Geometry: final body of the model. Coordinates: model frame, mm. A direction names the side the tool comes from. Give positions to 0.01 mm unless a question says otherwise; leave off trailing zeros. Order: outer loops, then holes, each group sorted by start corner. A loop starts at its lowest first (then second) coordinate and runs counter-clockwise, first axis right, second up. Notation, with made-up numbers: (-17.75, 41.25) - (35.25, 41.25) arc R19 cw to (35.25, 73.25) - close; hole circle Ø5 at (53, -5). An arc over 180 degrees is marked (long way). Use one line per item in the form item = value.
from build123d import *

# Parameters (mm, degrees)
SKETCH1_R           = 30
BOSS_EXTRUDE1_DEPTH = 2
SKETCH2_R           = 7.5
BOSS_EXTRUDE2_DEPTH = 7
BOSS_EXTRUDE3_DEPTH = 15
CUT_EXTRUDE1_DEPTH  = 18
CIRPATTERN2_COUNT   = 6


with BuildPart() as part:
    # Sketch1 → Boss-Extrude1 (new body)
    with BuildSketch(Plane(origin=(0, 0, 0), x_dir=(1, 0, 0), z_dir=(0, 1, 0))):
        Circle(SKETCH1_R)
    extrude(amount=BOSS_EXTRUDE1_DEPTH)

    # Sketch2 → Boss-Extrude2 (add)
    with BuildSketch(Plane(origin=(0, 0, 0), x_dir=(1, 0, 0), z_dir=(0, 1, 0))):
        Circle(SKETCH2_R)
    extrude(amount=BOSS_EXTRUDE2_DEPTH)

    # Sketch3 → Boss-Extrude3 (add)
    with BuildSketch(Plane(origin=(0, 2, 0), x_dir=(1, 0, 0), z_dir=(0, 1, 0))):
        with BuildLine():
            ThreePointArc((-27.399897799, 12.216611666), (-14.278250642, 14.389995002), (-3.458222056, 6.65512586))
            ThreePointArc((-3.458222056, 6.65512586), (-3.002192418, 6.872906277), (-2.532531954, 7.059481702))
            ThreePointArc((-2.532531954, 7.059481702), (-13.262608044, 15.162164286), (-26.638909527, 13.797409149))
            ThreePointArc((-26.638909527, 13.797409149), (-27.03096196, 13.012574516), (-27.399897799, 12.216611666))
        make_face()
        with BuildLine():
            ThreePointArc((-2.532531954, 7.059481702), (-2.038530942, 7.217644463), (-1.534779322, 7.341284113))
            ThreePointArc((-1.534779322, 7.341284113), (-12.178839524, 15.878170307), (-25.810761164, 15.290670625))
            ThreePointArc((-25.810761164, 15.290670625), (-26.235461619, 14.549933115), (-26.638909527, 13.797409149))
            ThreePointArc((-26.638909527, 13.797409149), (-13.262608044, 15.162164286), (-2.532531954, 7.059481702))
        make_face()
    boss_extrude3 = extrude(amount=BOSS_EXTRUDE3_DEPTH)

    # Sketch4 → Cut-Extrude1 (cut, through all)
    with BuildSketch(Plane(origin=(0, 0, 0), x_dir=(1, 0, 0), z_dir=(0, 1, 0))):
        with BuildLine():
            Line((-2.598076211, -1.5), (2.598076211, -1.5))
            ThreePointArc((2.598076211, -1.5), (0, 3), (-2.598076211, -1.5))
        make_face()
    extrude(amount=CUT_EXTRUDE1_DEPTH, mode=Mode.SUBTRACT)

    # CirPattern2: Boss-Extrude3 ×6 about axis
    cirpattern2_axis = Axis((0, 0, 0), (0, 1, 0))
    for i in range(1, CIRPATTERN2_COUNT):
        add(boss_extrude3.rotate(cirpattern2_axis, i * 360 / CIRPATTERN2_COUNT))


solid = part.part
(1) Reachability of faces 4 (the face through (13.6, 17, 14.4)), 5 (the face through (5.266, 9.395, -19.743)), 6 (the face through (0, 3, 1.5)) from +Z, -Z, +X, -X, +Y, -Y: full face, straight path, thin tool, end or side. Return the list, or none.
Computed values:
face_4 = +Z, -Z, +X, -X, +Y
face_5 = +Y
face_6 = +Y, -Y
(2) Pull-direction query (X, two-part tool) for faces 1 (the face through (-1.39, 4.46, 7.37)), 2 (the face through (-13.6, 17, -14.4)), 3 (the face through (19.694, 9.395, -2.479)); classes: released by +X, released by -X, zero draft, split by the parting line, or undercut.
Computed values:
face_1 = undercut
face_2 = zero draft
face_3 = released by +X
(3) Cut plane D-D on y = 15.25. Output: boundary loops of the cut face in (x, z).
Computed values:
outline = (-27.4, -12.22) arc R30 ccw to (-25.81, -15.29) arc R19.39 ccw to (-1.53, -7.34) arc R7.5 cw to (-3.46, -6.66) arc R17.39 cw to start; (-26.15, 14.71) arc R19.39 ccw to (-7.13, -2.34) arc R7.5 cw to (-7.49, -0.33) arc R17.39 cw to (-24.28, 17.62) arc R30 ccw to start; (-5.59, 5) arc R7.5 cw to (-4.03, 6.32) arc R17.39 cw to (3.12, 29.84) arc R30 ccw to (-0.34, 30) arc R19.39 ccw to start; (-3.12, -29.84) arc R30 ccw to (0.34, -30) arc R19.39 ccw to (5.59, -5) arc R7.5 cw to (4.03, -6.32) arc R17.39 cw to start; (1.53, 7.34) arc R7.5 cw to (3.46, 6.66) arc R17.39 cw to (27.4, 12.22) arc R30 ccw to (25.81, 15.29) arc R19.39 ccw to start; (7.13, 2.34) arc R7.5 cw to (7.49, 0.33) arc R17.39 cw to (24.28, -17.62) arc R30 ccw to (26.15, -14.71) arc R19.39 ccw to start
(4) Cut plane C-C on z = -23. Output: boundary loops of the cut face in (x, y).
Computed values:
outline = (-19.26, 0) - (19.26, 0) - (19.26, 2) - (6.11, 2) - (6.11, 17) - (3.86, 17) - (3.86, 2) - (-19.26, 2) - close
(5) Ray query, line 1 along Z through (x, y) = (0, 4.5); line 2 along Z through (x, y) = (0, 1.75); line 3 along Y through (x, z) = (5, 1). Return the intervals inside material, ascending.
Computed values:
line_1 = -30 to -27.7, -7.5 to -3, 1.5 to 7.5, 27.7 to 30
line_2 = -30 to -3, 1.5 to 30
line_3 = 0 to 7
(6) Contact query for flat-ended pins moving along their axis: pin 1 Ø3 at (y, z) = (6, 19.5) entering from -X; pin 2 Ø1.5 at (y, z) = (12, 2) entering from -X; pin 3 Ø3 at (y, z) = (14, 7.5) entering from +X. Output: stop coordinate, or through.
Computed values:
pin_1 = -7.76
pin_2 = -20
pin_3 = 5.21
(7) Cut plane B-B on x = -19. Output: boundary loops of the cut face in (y, z).
Computed values:
outline = (0, -23.22) - (2, -23.22) - (2, -16.83) - (17, -16.83) - (17, -14.82) - (2, -14.82) - (2, 1.9) - (17, 1.9) - (17, 4.56) - (2, 4.56) - (2, 23.22) - (0, 23.22) - close
(8) Cut plane A-A on y = 4.5. Output: boundary loops of the cut face in (x, z), plus the area to 3 significant figures.
Computed values:
outline = (-27.4, -12.22) arc R30 ccw to (-25.81, -15.29) arc R19.39 ccw to (-1.53, -7.34) arc R7.5 ccw to (4.03, -6.32) arc R17.39 cw to (-3.12, -29.84) arc R30 ccw to (0.34, -30) arc R19.39 ccw to (5.59, -5) arc R7.5 ccw to (7.49, 0.33) arc R17.39 cw to (24.28, -17.62) arc R30 ccw to (26.15, -14.71) arc R19.39 ccw to (7.13, 2.34) arc R7.5 ccw to (3.46, 6.66) arc R17.39 cw to (27.4, 12.22) arc R30 ccw to (25.81, 15.29) arc R19.39 ccw to (1.53, 7.34) arc R7.5 ccw to (-4.03, 6.32) arc R17.39 cw to (3.12, 29.84) arc R30 ccw to (-0.34, 30) arc R19.39 ccw to (-5.59, 5) arc R7.5 ccw to (-7.49, -0.33) arc R17.39 cw to (-24.28, 17.62) arc R30 ccw to (-26.15, 14.71) arc R19.39 ccw to (-7.13, -2.34) arc R7.5 ccw to (-3.46, -6.66) arc R17.39 cw to start; hole (-2.6, 1.5) arc R3 ccw (long way) to (2.6, 1.5) - close
area = 485 mm²
